```python
from build123d import *

# Parameters (mm, degrees)
BOSS_EXTRUDE1_DEPTH = 3.175
SKETCH2_R           = 1
CUT_EXTRUDE1_DEPTH  = 3.175
SKETCH3_W           = 3.175
SKETCH3_H           = 10.970571453
CUT_EXTRUDE2_DEPTH  = 48.905483945
SKETCH4_W           = 2
SKETCH4_H           = 2
CUT_EXTRUDE3_DEPTH  = 48.905483945


with BuildPart() as part:
    # Sketch1 → Boss-Extrude1 (new body)
    with BuildSketch(Plane.XY.offset(299.790013628)):
        with BuildLine():
            Line((33.800017398, -7.366761895), (33.800017398, 18.725816778))
            ThreePointArc((33.800017398, 18.725816778), (-0.000557823, 33.799609088), (-33.799982602, 18.723237361))
            Line((-33.799982602, 18.723237361), (-33.799982602, -7.366777732))
            add(Edge.make_bspline(
                [(-33.799982602, -7.366777732), (-33.672789327, -7.463259542), (-33.552121131, -7.566964097), (-33.326159842, -7.79139223), (-33.221125409, -7.912162508), (-33.034465703, -8.166471978), (-32.952054517, -8.300699067), (-32.811712114, -8.585009668), (-32.753980555, -8.735399478), (-32.711505515, -8.889768336)],
                knots=[0, 0, 0, 0, 0.25, 0.25, 0.5, 0.5, 0.75, 0.75, 1, 1, 1, 1], degree=3))
            add(Edge.make_bspline(
                [(-32.711505515, -8.889768336), (-32.218545569, -10.681353815), (-31.582970442, -12.406292143), (-30.046873209, -15.732353364), (-29.149732094, -17.335056266), (-27.853684449, -19.256830618), (-27.585876179, -19.636654103), (-27.037545067, -20.380994298), (-26.194235478, -21.477177142), (-25.289410486, -22.513279461), (-23.400136465, -24.507717332), (-22.036872596, -25.736014695), (-20.198644798, -27.140367507), (-19.823359112, -27.415057973), (-18.307010857, -28.47732838), (-17.130998838, -29.195842865), (-14.299650354, -30.696188469), (-12.615858618, -31.420604816), (-9.99268241, -32.310524634), (-9.099644071, -32.573674181), (-7.309378259, -33.021437293), (-4.607325738, -33.579354316), (-1.855822888, -33.799578534), (7.014e-06, -33.799609106)],
                knots=[0, 0, 0, 0, 0.125, 0.125, 0.25, 0.25, 0.28125, 0.28125, 0.3125, 0.375, 0.375, 0.5, 0.5, 0.53125, 0.53125, 0.625, 0.625, 0.75, 0.75, 0.8125, 0.8125, 0.875, 1, 1, 1, 1], degree=3))
            add(Edge.make_bspline(
                [(7.014e-06, -33.799609106), (3.71198449, -33.799546475), (7.323818522, -33.211894011), (11.272281305, -31.876901766), (11.709255106, -31.719210387), (12.572214597, -31.3883335), (13.853276296, -30.867912798), (16.748236975, -29.483886242), (19.066155809, -28.003005579), (20.904820016, -26.601476418), (21.26870544, -26.312112405), (21.981822477, -25.721047769), (22.331302421, -25.41922276), (23.359250005, -24.495530592), (25.333391288, -22.575468921), (27.05775769, -20.433363088), (28.609537919, -18.137832091), (29.098956145, -17.344856534), (30.005077972, -15.734456147), (30.424297285, -14.914397351), (31.581811664, -12.410251613), (32.218491785, -10.681549287), (32.711505515, -8.889768336)],
                knots=[0, 0, 0, 0, 0.25, 0.25, 0.28125, 0.28125, 0.3125, 0.375, 0.5, 0.5, 0.53125, 0.53125, 0.5625, 0.5625, 0.625, 0.75, 0.75, 0.8125, 0.8125, 0.875, 0.875, 1, 1, 1, 1], degree=3))
            add(Edge.make_bspline(
                [(32.711505515, -8.889768336), (32.79670017, -8.580141747), (32.939002514, -8.296331804), (33.317854255, -7.780583107), (33.545155986, -7.560077249), (33.800017398, -7.366761895)],
                knots=[0, 0, 0, 0, 0.5, 0.5, 1, 1, 1, 1], degree=3))
        make_face()
    extrude(amount=-BOSS_EXTRUDE1_DEPTH)

    # Sketch2 → Cut-Extrude1 (cut)
    with BuildSketch(Plane(origin=(0, 0, 296.615013628), x_dir=(-1, 0, 0), z_dir=(0, 0, -1))):
        with Locations((-32.009302375, -5.358989516)):
            Circle(SKETCH2_R)
        with Locations((31.216064399, -8.164436653)):
            Circle(SKETCH2_R)
    extrude(amount=-CUT_EXTRUDE1_DEPTH, mode=Mode.SUBTRACT)

    # Sketch3 → Cut-Extrude2 (cut, through all)
    with BuildSketch(Plane.XY.offset(299.790013628)):
        with Locations((-0.013127042, -29.284890239)):
            Rectangle(SKETCH3_W, SKETCH3_H)
    extrude(amount=-CUT_EXTRUDE2_DEPTH, mode=Mode.SUBTRACT)

    # Sketch4 → Cut-Extrude3 (cut, through all)
    with BuildSketch(Plane(origin=(0, 0, 296.615013628), x_dir=(-1, 0, 0), z_dir=(0, 0, -1))):
        with BuildLine():
            Line((14.257724699, -8.984256283), (14.257724699, 4.717183699))
            ThreePointArc((14.257724699, 4.717183699), (13.379045042, 6.838504042), (11.257724699, 7.717183699))
            Line((11.257724699, 7.717183699), (-14.878600613, 7.717183699))
            ThreePointArc((-14.878600613, 7.717183699), (-16.999920956, 6.838504042), (-17.878600613, 4.717183699))
            Line((-17.878600613, 4.717183699), (-17.878600613, -8.984256283))
            ThreePointArc((-17.878600613, -8.984256283), (-16.999920956, -11.105576627), (-14.878600613, -11.984256283))
            Line((-14.878600613, -11.984256283), (11.257724699, -11.984256283))
            ThreePointArc((11.257724699, -11.984256283), (13.379045042, -11.105576627), (14.257724699, -8.984256283))
        make_face()
        with Locations((15.257724699, -4.150157902)):
            Rectangle(SKETCH4_W, SKETCH4_H)
        with Locations((-18.878600613, -4.150157902)):
            Rectangle(SKETCH4_W, SKETCH4_H)
    extrude(amount=-CUT_EXTRUDE3_DEPTH, mode=Mode.SUBTRACT)


solid = part.part
```
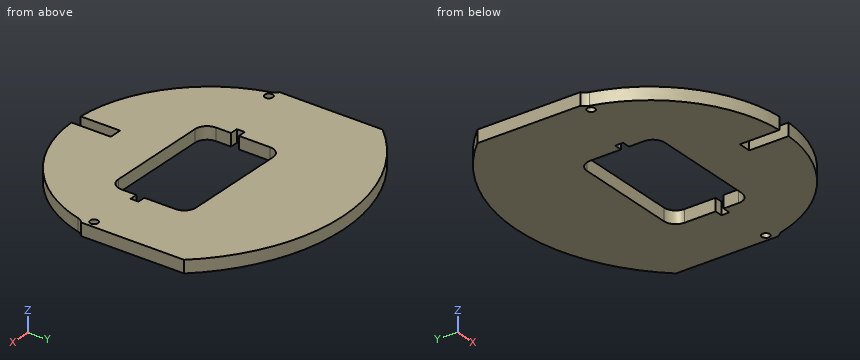
Work out the finished part from the listing and answer in its coordinate system (mm). Round coordinates to 2 decimals unless told otherwise and drop trailing zeros. Order: outer loops, then holes, each group sorted by start corner. A loop starts at its lowest first (then second) coordinate and runs counter-clockwise, first axis right, second up.
Q1. A cutting plane is placed at A-A, the plane y = 2.5. Determine the outline of the cut face in (x, z).
Solution:
outline: (-33.8, 296.62) - (-14.26, 296.62) - (-14.26, 299.79) - (-33.8, 299.79) - close; (17.88, 296.62) - (33.8, 296.62) - (33.8, 299.79) - (17.88, 299.79) - close
Q2. A cutting plane is placed at B-B, the plane z = 297.2. Count the separate pieces of the cut face and the enclosed holes in it, then the cut area to 3 significant figures.
Solution:
separate pieces: 1
enclosed holes: 3
area: 3,100 mm2
Q3. Find the intervals of material crossed by line 1 along X through (y, z) = (-5.5, 299.05); line 2 along Y through (x, z) = (8.5, 297.95); line 3 along Y through (x, z) = (-0.5, 296.9), in increasing order.
Solution:
line 1: x = -33.8 to -14.26, 17.88 to 31.02, 33 to 33.8
line 2: y = -32.72 to -11.98, 7.72 to 33
line 3: y = -23.8 to -11.98, 7.72 to 33.8
Q4. Given pin 1 Ø1.6 at (x, z) = (7.5, 297.5) entering from +Y; pin 2 Ø1.6 at (x, z) = (-15.5, 297.5) entering from -Y; pin 3 Ø1 at (y, z) = (-18, 299.5) entering from +X, each flat-ended and moving along its own axis, determine where each tip first touches the part or whether it passes through.
Solution:
pin 1: stops at y = 33.3
pin 2: stops at y = -30.45
pin 3: stops at x = 28.99
